Geometry check sheet. Reference: the model listing, model coordinates, mm. Face numbers are marked on the shaded views. A direction names the side the tool comes from. Round coordinates to 2 decimals unless told otherwise and drop trailing zeros. Order: outer loops, then holes, each group sorted by start corner. A loop starts at its lowest first (then second) coordinate and runs counter-clockwise, first axis right, second up. Notation, with made-up numbers: (68.5, 47.25) - (85.5, 47.25) arc R16 ccw to (85.5, 76.25) - close; hole circle Ø3 at (23.25, 12). An arc over 180 degrees is marked (long way). Return JSON: item names as keys, results as strings. Group by question number.
Q1. Tool access check on the marked faces 5 and 6. Record the directions out of +Z, -Z, +X, -X, +Y, -Y that give a thin tool (end or side, any length) a straight path to the whole face; none if there is none.
Q2. Sectioned sample at B-B, the plane x = -33. Record the cut outline in (y, z).
Q3. Draft check along X on the marked faces 1, 2, 3 and 4. Enter one of: pulls with the +X half, pulls with the -X half, needs draft (parallel to the pull), parting line crosses it, or undercut.
Q4. Sectioned sample at A-A, the plane y = -28.5. Record the cut outline in (x, z).
Q5. Gauge pin test, flat ends, axial feed: pin 1 Ø1 at (x, z) = (-13, -1.5) entering from -Y; pin 2 Ø5 at (x, y) = (19.375, -22.5) entering from -Z; pin 3 Ø6 at (x, y) = (19.375, -22.5) entering from +Z; pin 4 Ø4.5 at (x, y) = (-19.375, -22.5) entering from +Z. Record the tip position at first contact, or that the pin passes through.
Q6. Material ranges on line 1 along X through (y, z) = (-22.5, 7.45) (3 decimals); line 2 along Z through (x, y) = (33, -22); line 3 along X through (y, z) = (-12, -6.75), recorded low to high.
Q7. Sectioned sample at C-C, the plane y = -22.5. Give the number of separate pieces and of enclosed holes in the cut face, then the cut area to 3 significant figures.
```python
from build123d import *

# Parameters (mm, degrees)
SKETCH_W          = 80
SKETCH_H          = 19
PAD_DEPTH         = 45
SKETCH001_W       = 75
SKETCH001_H       = 14
POCKET_DEPTH      = 0.001
POCKET_DEPTH_BACK = 45.001
SKETCH002_R       = 3.75
POCKET001_DEPTH   = 3.5
SKETCH003_R       = 1.875
POCKET002_DEPTH   = 2.5
CHAMFER_SIZE      = 2.485
SKETCH004_W       = 80
SKETCH004_H       = 19
PAD001_DEPTH      = 2
FILLET_R          = 1


with BuildPart() as part:
    # Sketch → Pad (new body)
    with BuildSketch(Plane.XZ):
        Rectangle(SKETCH_W, SKETCH_H)
    extrude(amount=PAD_DEPTH)

    # Sketch001 → Pocket (cut, two sides)
    with BuildSketch(Plane.XZ) as pocket_sk:
        Rectangle(SKETCH001_W, SKETCH001_H)
    extrude(amount=-POCKET_DEPTH, mode=Mode.SUBTRACT)
    extrude(pocket_sk.sketch, amount=POCKET_DEPTH_BACK, mode=Mode.SUBTRACT)

    # Sketch002 (on DatumPlane) → Pocket001 (cut)
    with BuildSketch(Plane(origin=(0, 0, 9.5), x_dir=(-1, 0, 0), z_dir=(0, 0, 1))):
        with Locations((-19.375, 22.5)):
            Circle(SKETCH002_R)
        with Locations((19.375, 22.5)):
            Circle(SKETCH002_R)
    extrude(amount=-POCKET001_DEPTH, mode=Mode.SUBTRACT)

    # Sketch003 (on DatumPlane) → Pocket002 (cut)
    with BuildSketch(Plane(origin=(0, 0, -7), x_dir=(-1, 0, 0), z_dir=(0, 0, 1))):
        with Locations((-19.375, 22.5)):
            Circle(SKETCH003_R)
        with Locations((19.375, 22.5)):
            Circle(SKETCH003_R)
    extrude(amount=-POCKET002_DEPTH, mode=Mode.SUBTRACT)

    # Chamfer
    chamfer_edges = [part.edges().sort_by_distance(p)[0] for p in [
        (-17.5, -22.5, -7),
        (21.25, -22.5, -7),
    ]]
    chamfer(chamfer_edges, length=CHAMFER_SIZE)

    # Sketch004 → Pad001 (join)
    with BuildSketch(Plane.XZ):
        Rectangle(SKETCH004_W, SKETCH004_H)
    extrude(amount=PAD001_DEPTH)

    # Fillet
    fillet_edges = [part.edges().sort_by_distance(p)[0] for p in [
        (-40, -45, 0),
        (0, -45, 9.5),
        (0, -45, -9.5),
        (40, -45, 0),
        (-37.5, -45, 0),
        (0, -45, 7),
        (37.5, -45, 0),
        (0, -45, -7),
        (40, -23.5, 9.5),
        (40, -23.5, -9.5),
        (-40, -23.5, 9.5),
        (-40, -23.5, -9.5),
        (0, 0, 9.5),
        (-40, 0, 0),
        (40, 0, 0),
        (40, -1, 9.5),
        (-40, -1, 9.5),
        (-40, -1, -9.5),
        (40, -1, -9.5),
        (0, 0, -9.5),
        (-15.625, -22.5, 9.5),
        (23.125, -22.5, 9.5),
    ]]
    fillet(fillet_edges, radius=FILLET_R)


solid = part.part
```
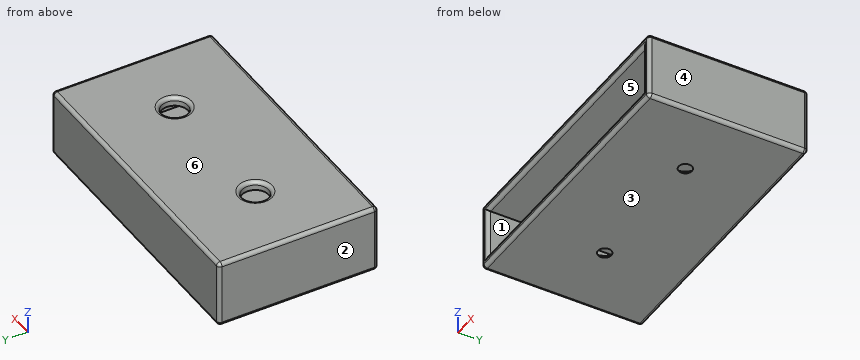
Reply:
{
 "1": {"face 5": "-Y", "face 6": "+Z, +X, -X, +Y, -Y"},
 "2": {"outline": "(-45, -8.5) arc R1 ccw to (-44, -9.5) - (-1, -9.5) arc R1 ccw to (0, -8.5) - (0, 8.5) arc R1 ccw to (-1, 9.5) - (-44, 9.5) arc R1 ccw to (-45, 8.5) - (-45, 8) arc R1 ccw to (-44, 7) - (-2, 7) - (-2, -7) - (-44, -7) arc R1 ccw to (-45, -8) - close"},
 "3": {"face 1": "undercut", "face 2": "pulls with the -X half", "face 3": "needs draft", "face 4": "pulls with the +X half"},
 "4": {"outline": "(-40, -8.5) arc R1 ccw to (-39, -9.5) - (39, -9.5) arc R1 ccw to (40, -8.5) - (40, 8.5) arc R1 ccw to (39, 9.5) - (-39, 9.5) arc R1 ccw to (-40, 8.5) - close; hole (-37.5, -7) - (37.5, -7) - (37.5, 7) - (-37.5, 7) - close"},
 "5": {"pin 1": "y = -2", "pin 2": "z = -9.5", "pin 3": "z = -8.36", "pin 4": "z = -9.11"},
 "6": {"line 1": "-40 to -23.125, -15.625 to 15.625, 23.125 to 40", "line 2": "-9.5 to -7, 7 to 9.5", "line 3": "-40 to -37.5, 37.5 to 40"},
 "7": {"separate pieces": "4", "enclosed holes": "0", "area": "400 mm^2"}
}
